Input: part model. Units: mm. Frame: model coordinates. Face numbers are marked on the shaded views. Give positions to 0.01 mm unless a question says otherwise; leave off trailing zeros. Loops run counter-clockwise (first coordinate to the right, second up) from the corner with the lowest first, then second, coordinate; pieces in that order, holes last. Notation, with made-up numbers: M 28,15 L 82,15 A21 ccw 82,40 Z; hole C 67,7.5 d11. An arc over 180 degrees is marked long. Answer as a JSON object with one key per item and string values. Group by question number.
```python
from build123d import *

# Parameters (mm, degrees)
BOSS_EXTRUDE1_DEPTH     = 3
FILLET4_R               = 8
FILLET5_R               = 3
SKETCH4_R               = 10
BOSS_EXTRUDE4_DEPTH     = 60
CHAMFER2_SIZE           = 17
CHAMFER2_SIZE2          = 42.076476508
FILLET7_R               = 4
SKETCH5_R               = 15
CUT_EXTRUDE1_DEPTH      = 32
FILLET8_R               = 3
SKETCH6_R               = 8.43
CUT_EXTRUDE2_DEPTH      = 15
FILLET9_R               = 4
CUT_EXTRUDE3_DEPTH      = 15
CUT_EXTRUDE3_DEPTH_BACK = 15


with BuildPart() as part:
    # Sketch1 → Boss-Extrude1 (new body)
    with BuildSketch(Plane(origin=(0, 0, 0), x_dir=(1, 0, 0), z_dir=(0, 1, 0))):
        with BuildLine():
            ThreePointArc((29.158991571, 15), (31.870032918, 7.716721534), (32.790955909, 0))
            Line((32.790955909, 0), (95, 0))
            Line((95, 0), (95, 15))
            Line((95, 15), (29.158991571, 15))
        make_face()
        with BuildLine():
            Line((95, 0), (32.790955909, 0))
            ThreePointArc((32.790955909, 0), (31.870032918, -7.716721534), (29.158991571, -15))
            Line((29.158991571, -15), (95, -15))
            Line((95, -15), (95, 0))
        make_face()
        with BuildLine():
            ThreePointArc((15, 29.158991571), (7.716721534, 31.870032918), (0, 32.790955909))
            Line((0, 32.790955909), (0, 0))
            Line((0, 0), (32.790955909, 0))
            ThreePointArc((32.790955909, 0), (31.870032918, 7.716721534), (29.158991571, 15))
            ThreePointArc((29.158991571, 15), (23.186707285, 23.186707285), (15, 29.158991571))
        make_face()
        with BuildLine():
            Line((0, 0), (0, 32.790955909))
            ThreePointArc((0, 32.790955909), (-7.716721534, 31.870032918), (-15, 29.158991571))
            ThreePointArc((-15, 29.158991571), (-23.186707285, 23.186707285), (-29.158991571, 15))
            ThreePointArc((-29.158991571, 15), (-31.870032918, 7.716721534), (-32.790955909, 0))
            Line((-32.790955909, 0), (0, 0))
        make_face()
        with BuildLine():
            Line((32.790955909, 0), (0, 0))
            Line((0, 0), (0, -32.790955909))
            ThreePointArc((0, -32.790955909), (7.716721534, -31.870032918), (15, -29.158991571))
            ThreePointArc((15, -29.158991571), (23.186707285, -23.186707285), (29.158991571, -15))
            ThreePointArc((29.158991571, -15), (31.870032918, -7.716721534), (32.790955909, 0))
        make_face()
        with BuildLine():
            Line((0, -32.790955909), (0, 0))
            Line((0, 0), (-32.790955909, 0))
            ThreePointArc((-32.790955909, 0), (-31.870032918, -7.716721534), (-29.158991571, -15))
            ThreePointArc((-29.158991571, -15), (-23.186707285, -23.186707285), (-15, -29.158991571))
            ThreePointArc((-15, -29.158991571), (-7.716721534, -31.870032918), (0, -32.790955909))
        make_face()
        with BuildLine():
            ThreePointArc((15, 29.158991571), (7.716721534, 31.870032918), (0, 32.790955909))
            Line((0, 32.790955909), (0, 0))
            Line((0, 0), (32.790955909, 0))
            ThreePointArc((32.790955909, 0), (31.870032918, 7.716721534), (29.158991571, 15))
            ThreePointArc((29.158991571, 15), (23.186707285, 23.186707285), (15, 29.158991571))
        make_face()
        with BuildLine():
            Line((0, 0), (0, 32.790955909))
            ThreePointArc((0, 32.790955909), (-7.716721534, 31.870032918), (-15, 29.158991571))
            ThreePointArc((-15, 29.158991571), (-23.186707285, 23.186707285), (-29.158991571, 15))
            ThreePointArc((-29.158991571, 15), (-31.870032918, 7.716721534), (-32.790955909, 0))
            Line((-32.790955909, 0), (0, 0))
        make_face()
        with BuildLine():
            Line((32.790955909, 0), (0, 0))
            Line((0, 0), (0, -32.790955909))
            ThreePointArc((0, -32.790955909), (7.716721534, -31.870032918), (15, -29.158991571))
            ThreePointArc((15, -29.158991571), (23.186707285, -23.186707285), (29.158991571, -15))
            ThreePointArc((29.158991571, -15), (31.870032918, -7.716721534), (32.790955909, 0))
        make_face()
        with BuildLine():
            Line((0, -32.790955909), (0, 0))
            Line((0, 0), (-32.790955909, 0))
            ThreePointArc((-32.790955909, 0), (-31.870032918, -7.716721534), (-29.158991571, -15))
            ThreePointArc((-29.158991571, -15), (-23.186707285, -23.186707285), (-15, -29.158991571))
            ThreePointArc((-15, -29.158991571), (-7.716721534, -31.870032918), (0, -32.790955909))
        make_face()
        with BuildLine():
            ThreePointArc((15, 29.158991571), (7.716721534, 31.870032918), (0, 32.790955909))
            Line((0, 32.790955909), (0, 0))
            Line((0, 0), (32.790955909, 0))
            ThreePointArc((32.790955909, 0), (31.870032918, 7.716721534), (29.158991571, 15))
            ThreePointArc((29.158991571, 15), (23.186707285, 23.186707285), (15, 29.158991571))
        make_face()
        with BuildLine():
            Line((0, 0), (0, 32.790955909))
            ThreePointArc((0, 32.790955909), (-7.716721534, 31.870032918), (-15, 29.158991571))
            ThreePointArc((-15, 29.158991571), (-23.186707285, 23.186707285), (-29.158991571, 15))
            ThreePointArc((-29.158991571, 15), (-31.870032918, 7.716721534), (-32.790955909, 0))
            Line((-32.790955909, 0), (0, 0))
        make_face()
        with BuildLine():
            Line((32.790955909, 0), (0, 0))
            Line((0, 0), (0, -32.790955909))
            ThreePointArc((0, -32.790955909), (7.716721534, -31.870032918), (15, -29.158991571))
            ThreePointArc((15, -29.158991571), (23.186707285, -23.186707285), (29.158991571, -15))
            ThreePointArc((29.158991571, -15), (31.870032918, -7.716721534), (32.790955909, 0))
        make_face()
        with BuildLine():
            Line((0, -32.790955909), (0, 0))
            Line((0, 0), (-32.790955909, 0))
            ThreePointArc((-32.790955909, 0), (-31.870032918, -7.716721534), (-29.158991571, -15))
            ThreePointArc((-29.158991571, -15), (-23.186707285, -23.186707285), (-15, -29.158991571))
            ThreePointArc((-15, -29.158991571), (-7.716721534, -31.870032918), (0, -32.790955909))
        make_face()
        with BuildLine():
            ThreePointArc((15, 29.158991571), (7.716721534, 31.870032918), (0, 32.790955909))
            Line((0, 32.790955909), (0, 0))
            Line((0, 0), (32.790955909, 0))
            ThreePointArc((32.790955909, 0), (31.870032918, 7.716721534), (29.158991571, 15))
            ThreePointArc((29.158991571, 15), (23.186707285, 23.186707285), (15, 29.158991571))
        make_face()
        with BuildLine():
            Line((0, 0), (0, 32.790955909))
            ThreePointArc((0, 32.790955909), (-7.716721534, 31.870032918), (-15, 29.158991571))
            ThreePointArc((-15, 29.158991571), (-23.186707285, 23.186707285), (-29.158991571, 15))
            ThreePointArc((-29.158991571, 15), (-31.870032918, 7.716721534), (-32.790955909, 0))
            Line((-32.790955909, 0), (0, 0))
        make_face()
        with BuildLine():
            Line((32.790955909, 0), (0, 0))
            Line((0, 0), (0, -32.790955909))
            ThreePointArc((0, -32.790955909), (7.716721534, -31.870032918), (15, -29.158991571))
            ThreePointArc((15, -29.158991571), (23.186707285, -23.186707285), (29.158991571, -15))
            ThreePointArc((29.158991571, -15), (31.870032918, -7.716721534), (32.790955909, 0))
        make_face()
        with BuildLine():
            Line((0, -32.790955909), (0, 0))
            Line((0, 0), (-32.790955909, 0))
            ThreePointArc((-32.790955909, 0), (-31.870032918, -7.716721534), (-29.158991571, -15))
            ThreePointArc((-29.158991571, -15), (-23.186707285, -23.186707285), (-15, -29.158991571))
            ThreePointArc((-15, -29.158991571), (-7.716721534, -31.870032918), (0, -32.790955909))
        make_face()
        with BuildLine():
            Line((0, 32.790955909), (0, 95))
            Line((0, 95), (-15, 95))
            Line((-15, 95), (-15, 29.158991571))
            ThreePointArc((-15, 29.158991571), (-7.716721534, 31.870032918), (0, 32.790955909))
        make_face()
        with BuildLine():
            Line((15, 95), (0, 95))
            Line((0, 95), (0, 32.790955909))
            ThreePointArc((0, 32.790955909), (7.716721534, 31.870032918), (15, 29.158991571))
            Line((15, 29.158991571), (15, 95))
        make_face()
        with BuildLine():
            Line((-95, 0), (-32.790955909, 0))
            ThreePointArc((-32.790955909, 0), (-31.870032918, 7.716721534), (-29.158991571, 15))
            Line((-29.158991571, 15), (-95, 15))
            Line((-95, 15), (-95, 0))
        make_face()
        with BuildLine():
            ThreePointArc((-29.158991571, -15), (-31.870032918, -7.716721534), (-32.790955909, 0))
            Line((-32.790955909, 0), (-95, 0))
            Line((-95, 0), (-95, -15))
            Line((-95, -15), (-29.158991571, -15))
        make_face()
        with BuildLine():
            Line((0, -95), (0, -32.790955909))
            ThreePointArc((0, -32.790955909), (-7.716721534, -31.870032918), (-15, -29.158991571))
            Line((-15, -29.158991571), (-15, -95))
            Line((-15, -95), (0, -95))
        make_face()
        with BuildLine():
            ThreePointArc((15, -29.158991571), (7.716721534, -31.870032918), (0, -32.790955909))
            Line((0, -32.790955909), (0, -95))
            Line((0, -95), (15, -95))
            Line((15, -95), (15, -29.158991571))
        make_face()
    extrude(amount=BOSS_EXTRUDE1_DEPTH)

    # Fillet4
    fillet4_edges = [part.edges().sort_by_distance(p)[0] for p in [
        (95, 1.5, -15),
        (95, 1.5, 15),
        (15, 1.5, 95),
        (-15, 1.5, 95),
        (-95, 1.5, 15),
        (-95, 1.5, -15),
        (-15, 1.5, -95),
        (15, 1.5, -95),
    ]]
    fillet(fillet4_edges, radius=FILLET4_R)

    # Fillet5
    fillet5_edges = [part.edges().sort_by_distance(p)[0] for p in [
        (-12.656854249, 3, 92.656854249),
        (-15, 3, 58.079495785),
        (-23.186707285, 3, 23.186707285),
        (-58.079495785, 3, 15),
        (-92.656854249, 3, 12.656854249),
        (-95, 3, 0),
        (-92.656854249, 3, -12.656854249),
        (-58.079495785, 3, -15),
        (-23.186707285, 3, -23.186707285),
        (-15, 3, -58.079495785),
        (-12.656854249, 3, -92.656854249),
        (0, 3, -95),
        (12.656854249, 3, -92.656854249),
        (15, 3, -58.079495785),
        (23.186707285, 3, -23.186707285),
        (58.079495785, 3, -15),
        (92.656854249, 3, -12.656854249),
        (95, 3, 0),
        (92.656854249, 3, 12.656854249),
        (58.079495785, 3, 15),
        (23.186707285, 3, 23.186707285),
        (15, 3, 58.079495785),
        (12.656854249, 3, 92.656854249),
        (0, 3, 95),
    ]]
    fillet(fillet5_edges, radius=FILLET5_R - 0.0001)  # a hair under: the kernel refuses the full size

    # Sketch4 → Boss-Extrude4 (add)
    with BuildSketch(Plane(origin=(0, 3, 0), x_dir=(1, 0, 0), z_dir=(0, 1, 0))):
        with Locations(Location((0, 0, 0), (0, 0, 270))):
            Circle(SKETCH4_R)
    extrude(amount=BOSS_EXTRUDE4_DEPTH)

    # Chamfer2
    chamfer2_edges = [part.edges().sort_by_distance(p)[0] for p in [
        (0, 3, -10),
    ]]
    chamfer2_side = [part.faces().sort_by_distance(p)[0] for p in [
        (9.397944217, 3, 57.133640491),
    ]]
    chamfer(chamfer2_edges, length=CHAMFER2_SIZE, length2=CHAMFER2_SIZE2, reference=chamfer2_side[0])

    # Fillet7
    fillet7_edges = [part.edges().sort_by_distance(p)[0] for p in [
        (0, 45.076476508, -10),
    ]]
    fillet(fillet7_edges, radius=FILLET7_R)

    # Sketch5 → Cut-Extrude1 (cut)
    with BuildSketch(Plane.XZ):
        with Locations(Location((0, 0, 0), (0, 0, 270))):
            Circle(SKETCH5_R)
    extrude(amount=-CUT_EXTRUDE1_DEPTH, mode=Mode.SUBTRACT)

    # Fillet8
    fillet8_edges = [part.edges().sort_by_distance(p)[0] for p in [
        (0, 3, -27),
    ]]
    fillet(fillet8_edges, radius=FILLET8_R)

    # Sketch6 → Cut-Extrude2 (cut)
    with BuildSketch(Plane(origin=(0, 63, 0), x_dir=(1, 0, 0), z_dir=(0, 1, 0))):
        with Locations(Location((0, 0, 0), (0, 0, 270))):
            Circle(SKETCH6_R)
    extrude(amount=-CUT_EXTRUDE2_DEPTH, mode=Mode.SUBTRACT)

    # Fillet9
    fillet9_edges = [part.edges().sort_by_distance(p)[0] for p in [
        (0, 32, 15),
    ]]
    fillet(fillet9_edges, radius=FILLET9_R)

    # Sketch8 → Cut-Extrude3 (cut, two sides: drawn at the far end of the back side and taken through both)
    with BuildSketch(Plane(origin=(0, 0, 0), x_dir=(0, 0, -1), z_dir=(1, 0, 0)).offset(-CUT_EXTRUDE3_DEPTH_BACK)):
        with BuildLine():
            Line((0, 55.5), (0, 57.1))
            ThreePointArc((0, 57.1), (-1.6, 55.5), (0, 53.9))
            Line((0, 53.9), (0, 55.5))
        make_face()
        with BuildLine():
            ThreePointArc((1.6, 55.5), (1.13137085, 56.63137085), (0, 57.1))
            Line((0, 57.1), (0, 55.5))
            Line((0, 55.5), (1.6, 55.5))
        make_face()
        with BuildLine():
            Line((1.6, 55.5), (0, 55.5))
            Line((0, 55.5), (0, 53.9))
            ThreePointArc((0, 53.9), (1.13137085, 54.36862915), (1.6, 55.5))
        make_face()
        with BuildLine():
            ThreePointArc((1.6, 55.5), (1.13137085, 56.63137085), (0, 57.1))
            Line((0, 57.1), (0, 55.5))
            Line((0, 55.5), (1.6, 55.5))
        make_face()
        with BuildLine():
            Line((1.6, 55.5), (0, 55.5))
            Line((0, 55.5), (0, 53.9))
            ThreePointArc((0, 53.9), (1.13137085, 54.36862915), (1.6, 55.5))
        make_face()
    extrude(amount=CUT_EXTRUDE3_DEPTH + CUT_EXTRUDE3_DEPTH_BACK, mode=Mode.SUBTRACT)


solid = part.part
```
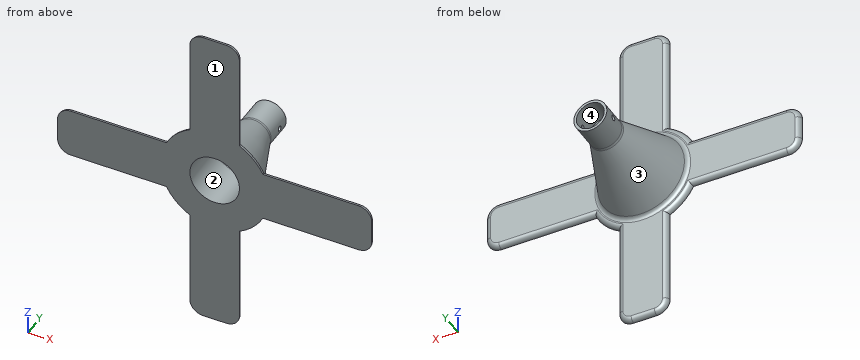
1. First-contact query: P1, Ø12, axis at y = 43, z = -10.5, coming from the +X side; P2, Ø1, axis at y = 17, z = -16, coming from the +X side; P3, Ø15, axis at x = 0, z = 0, coming from the +Y side. Flat tips, straight axial feed; report the tip coordinate or a pass-through.
2. Mould query, pull axis Z, two halves, no side actions, for the marked faces 1, 2, 3 and 4. Classes: pulls with the +Z half, pulls with the -Z half, needs draft (parallel to the pull), parting line crosses it, or undercut.
3. Material intervals for L1, parallel to X at y = 22, z = 0; L2, parallel to X at y = 52, z = 0; L3, parallel to X at y = 34, z = -9.5, sorted ascending.
4. Section C-C (y = 35). Output: boundary loops of the cut face in (x, z).
Geometry results:
{
 "1": {"P1": "x = 10.9", "P2": "x = 14.75", "P3": "y = 48"},
 "2": {"face 1": "needs draft", "face 2": "undercut", "face 3": "parting line crosses it", "face 4": "undercut"},
 "3": {"L1": "-19.32 to -15, 15 to 19.32", "L2": "-10 to -8.43, 8.43 to 10", "L3": "-10.92 to 10.92"},
 "4": {"outline": "C 0,0 d28.14"}
}
